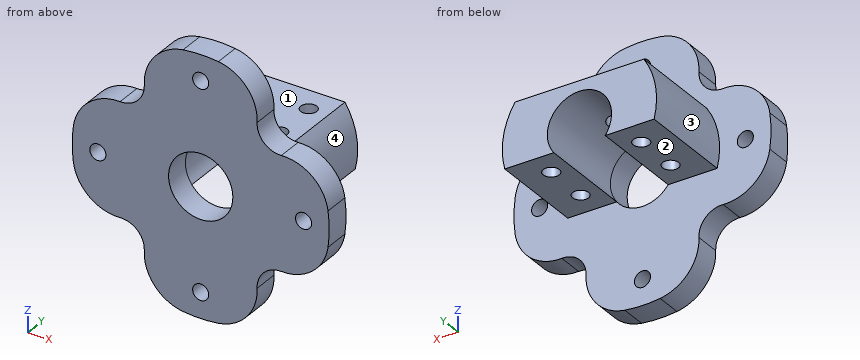
from build123d import *
from build123d.topology import SkipClean

# Parameters (mm, degrees)
EXTRUDE_1_DEPTH     = 15
EXTRUDE_START       = -4
SKETCH_3_R          = 20
SKETCH_3_R_2        = 1.25
SKETCH_3_R_3        = 5
EXTRUDE_2_DEPTH     = 4
SKETCH_4_R          = 3.6
CUT_EXTRUDE_1_DEPTH = 33.015621
FILLET_1_R          = 7
SKETCH_5_R          = 1.25
SKETCH_5_R_2        = 1.5
CUT_EXTRUDE_2_DEPTH = 34.970576


with BuildPart() as part:
    # 草图2 → 凸台-拉伸1 (new body)
    with BuildSketch(Plane(origin=(0, 0, 0), x_dir=(1, 0, 0), z_dir=(0, 1, 0))):
        with BuildLine():
            Line((-10.021976, -6.6), (10.021976, -6.6))
            ThreePointArc((10.021976, -6.6), (11.837332, -1.969158), (11.61895, 3))
            Line((11.61895, 3), (4, 3))
            ThreePointArc((4, 3), (0, -5), (-4, 3))
            Line((-4, 3), (-11.61895, 3))
            ThreePointArc((-11.61895, 3), (-11.837332, -1.969158), (-10.021976, -6.6))
        make_face()
    extrude(amount=EXTRUDE_1_DEPTH)

    # 草图3 → 凸台-拉伸2 (add)
    with SkipClean():  # the faces are left unmerged after this step: merging them gives an invalid solid
        with BuildSketch(Plane(origin=(0, 0, 0), x_dir=(1, 0, 0), z_dir=(0, 1, 0)).offset(EXTRUDE_START)):
            with Locations(Location((0, 0, 0), (0, 0, 270))):
                Circle(SKETCH_3_R)
            with Locations(Location((0, -16, 0), (0, 0, 270))):
                Circle(SKETCH_3_R_2, mode=Mode.SUBTRACT)
            with Locations(Location((16, 0, 0), (0, 0, 270))):
                Circle(SKETCH_3_R_2, mode=Mode.SUBTRACT)
            with Locations(Location((-16, 0, 0), (0, 0, 270))):
                Circle(SKETCH_3_R_2, mode=Mode.SUBTRACT)
            with Locations(Location((0, 16, 0), (0, 0, 270))):
                Circle(SKETCH_3_R_2, mode=Mode.SUBTRACT)
            with Locations(Location((0, 0, 0), (0, 0, 143.130102))):
                Circle(SKETCH_3_R_3, mode=Mode.SUBTRACT)
        extrude(amount=EXTRUDE_2_DEPTH)

    # 草图4 → 切除-拉伸1 (cut, through all)
    with SkipClean():  # the faces are left unmerged after this step: merging them gives an invalid solid
        with BuildSketch(Plane(origin=(0, 0, 0), x_dir=(1, 0, 0), z_dir=(0, 1, 0))):
            with Locations((12.374369, -12.374369)):
                Circle(SKETCH_4_R)
            with Locations((12.374369, 12.374369)):
                Circle(SKETCH_4_R)
            with Locations((-12.374369, 12.374369)):
                Circle(SKETCH_4_R)
            with Locations((-12.374369, -12.374369)):
                Circle(SKETCH_4_R)
        extrude(amount=-CUT_EXTRUDE_1_DEPTH, mode=Mode.SUBTRACT)

    # 圆角1
    fillet_1_edges = [part.edges().sort_by_distance(p)[0] for p in [
        (-12.053138, -2, 15.960008),
        (-15.960008, -2, 12.053138),
        (-15.960008, -2, -12.053138),
        (-12.053138, -2, -15.960008),
        (12.053138, -2, -15.960008),
        (15.960008, -2, -12.053138),
        (15.960008, -2, 12.053138),
        (12.053138, -2, 15.960008),
    ]]
    fillet(fillet_1_edges, radius=FILLET_1_R)

    # 草图5 → 切除-拉伸2 (cut, through all)
    with SkipClean():  # the faces are left unmerged after this step: merging them gives an invalid solid
        with BuildSketch(Plane(origin=(0, 0, -3), x_dir=(-1, 0, 0), z_dir=(0, 0, -1))):
            with Locations((-7, 11)):
                Circle(SKETCH_5_R)
            with Locations((-7, 4)):
                Circle(SKETCH_5_R)
            with Locations((7, 11)):
                Circle(SKETCH_5_R)
            with Locations((7, 4)):
                Circle(SKETCH_5_R)
            with Locations((0, 6)):
                Circle(SKETCH_5_R_2)
        extrude(amount=-CUT_EXTRUDE_2_DEPTH, mode=Mode.SUBTRACT)


solid = part.part
Model file for the job. Use its own axes, mm. Face numbers are marked on the shaded views. A direction names the side the tool comes from. Coordinates: 2 decimals unless noted, no trailing zeros. Order: outer loops, then holes, each group sorted by start corner. A loop starts at its lowest first (then second) coordinate and runs counter-clockwise, first axis right, second up. Notation, with made-up numbers: M 82.5,67 L 92.5,67 A12 ccw 92.5,78 Z; hole C 0.25,-35.75 d5. An arc over 180 degrees is marked long. Return JSON: item names as keys, results as strings.
1. Flat gauge pins, fed straight in: pin 1 (10 mm diameter, centred on y = 9.5, z = -5, fed in from +X); pin 2 (4.5 mm diameter, centred on x = 3.5, y = 4, fed in from +Z); pin 3 (3 mm diameter, centred on x = -16, z = 0, fed in from -Y); pin 4 (2 mm diameter, centred on x = -14, y = -2, fed in from -Z). Where does each tip first touch, or does it go through?
Ans:
{"pin 1": "x = 12", "pin 2": "z = 6.6", "pin 3": "y = -4", "pin 4": "z = -8.79"}
2. Saw through at D-D (y = 6.5). Give the cut face in (x, z), and give its area (3 significant figures).
Ans:
{"outline": "M -11.62,-3 L -4,-3 A5 cw -1.41,4.8 L -1.41,6.6 L -10.02,6.6 A12 ccw Z; M 1.41,4.8 A5 cw 4,-3 L 11.62,-3 A12 ccw 10.02,6.6 L 1.41,6.6 Z", "area": "149 mm^2"}
3. Saw through at A-A (z = 0). Give the cut face in (x, y).
Ans:
{"outline": "M -20,-4 L -17.25,-4 L -17.25,0 L -20,0 Z; M -14.75,-4 L -5,-4 L -5,15 L -12,15 L -12,0 L -14.75,0 Z; M 5,-4 L 14.75,-4 L 14.75,0 L 12,0 L 12,15 L 5,15 Z; M 17.25,-4 L 20,-4 L 20,0 L 17.25,0 Z; hole C -7,4 d2.5; hole C -7,11 d2.5; hole C 7,4 d2.5; hole C 7,11 d2.5"}
4. Saw through at B-B (y = 4). Give the cut face in (x, z), and give its area (3 significant figures).
Ans:
{"outline": "M -11.62,-3 L -8.25,-3 L -8.25,6.6 L -10.02,6.6 A12 ccw Z; M -5.75,-3 L -4,-3 A5 cw long 4,-3 L 5.75,-3 L 5.75,6.6 L -5.75,6.6 Z; M 8.25,-3 L 11.62,-3 A12 ccw 10.02,6.6 L 8.25,6.6 Z", "area": "106 mm^2"}
5. Saw through at C-C (x = 0). Give the cut face in (y, z).
Ans:
{"outline": "M -4,-20 L 0,-20 L 0,-17.25 L -4,-17.25 Z; M -4,-14.75 L 0,-14.75 L 0,-5 L -4,-5 Z; M -4,5 L 4.5,5 L 4.5,6.6 L 0,6.6 L 0,14.75 L -4,14.75 Z; M -4,17.25 L 0,17.25 L 0,20 L -4,20 Z; M 7.5,5 L 15,5 L 15,6.6 L 7.5,6.6 Z"}
6. Tool access for the marked faces 1, 2, 3 and 4: list every direction of +Z, -Z, +X, -X, +Y, -Y with a clear straight run to the whole face (end or side of a thin tool).
Ans:
{"face 1": "+Z, +X, -X, +Y", "face 2": "-Z, +X, -X, +Y", "face 3": "-X, +Y", "face 4": "+X, +Y"}
7. Drill centre lines: probe 1 along X at (y, z) = (-1.8, 0); probe 2 along Y at (x, z) = (7, 2); probe 3 along Y at (x, z) = (-14, 2). Where is each one in solid material? Low to high.
Ans:
{"probe 1": "-20 to -17.25, -14.75 to -5, 5 to 14.75, 17.25 to 20", "probe 2": "-4 to 2.75, 5.25 to 9.75, 12.25 to 15", "probe 3": "-4 to 0"}
